Could you check a few things on this model? Use its own coordinates, in mm. A direction names the side the tool comes from. Give positions to 0.01 mm unless a question says otherwise; leave off trailing zeros. Order: outer loops, then holes, each group sorted by start corner. A loop starts at its lowest first (then second) coordinate and runs counter-clockwise, first axis right, second up. Notation, with made-up numbers: (-3.75, 35) -> (30.25, 35) arc R25 cw to (30.25, 58) -> close; hole circle Ø1 at (80.25, 31). An arc over 180 degrees is marked (long way). Write each question's results on one line, items separated by ' | '.
Autodesk Inventor part; units mm, degrees
ref_plane "YZ Plane" through (0, 0, 0) normal (1, 0, 0) x (0, 1, 0)
ref_plane "XZ Plane" through (0, 0, 0) normal (0, 1, 0) x (-1, 0, 0)
ref_plane "XY Plane" through (0, 0, 0) normal (0, 0, 1) x (1, 0, 0)
sketch "Esboço1" plane through (0, 0, 0) normal (0, 0, 1) x (1, 0, 0)
  circle A0 centre (0, 0) radius 10
  dimension "d0" = 20
extrude "Extrusão1" add sketch "Esboço1" along normal blind 38
chamfer "Chanfro1" distance 3 angle 45 1 edges at (-10, 0, 0)
sketch "Esboço3" plane through (0, 0, 0) normal (0, 1, 0) x (-1, 0, 0)
  line L0 (10, 38) -> (-10, 38)
  arc A0 (14.87, 38) -> (-14.87, 38) centre (0, 38) ccw
  line L1 (0, 52.87) -> (0, 38)
  line L2 (-14.87, 38) -> (14.87, 38)
  point P0 (0, 0)
  dimension "d7" = 29.74
revolve "Revolução1" add sketch "Esboço3" angle 360 about axis through (0, 0, 52.87) along (0, 0, -1) picked at (-6.4238, 41.8753) contours L0 L2 A0 L1
sketch "Esboço4" plane through (0, 0, 0) normal (0, 1, 0) x (-1, 0, 0)
  line L0 (-2, 57) -> (2, 57)
  line L1 (2, 57) -> (2, 41)
  line L2 (2, 41) -> (-2, 41)
  line L3 (-2, 41) -> (-2, 57)
  line L4 (7, 0) -> (-7, 0)
  point P0 (0, 0)
  point P1 (0, 0)
  dimension "d9" = 4
  dimension "d10" = 16
  dimension "d11" = 41
  dimension "d13" = 2
extrude "Extrusão2" cut sketch "Esboço4" along normal mid plane 38
properties part number "Parafuso da Valvula"
Q1. I need wall thicknesses on line 1 along Z through (x, y) = (1.5, 10.25); line 2 along Z through (x, y) = (-1, -5.75); line 3 along X through (y, z) = (4.25, 46.5). Which ranges of each line are inside material? Lowest first, please.
Here are the results:
line 1: z = 38 to 41 | line 2: z = 0 to 41 | line 3: x = -11.44 to -2, 2 to 11.44
Q2. Suppose I cut it at C-C on z = 6.5. Please give me the cut outline in (x, y).
Here are the results:
outline: circle Ø20 at (0, 0)
Q3. Thinking about a two-plate mould opening in X: for faces 4 (the conical face through (-1.56, -7.02, 0.19)), 5 (the flat face through (3, 10, 38)), 6 (the flat face through (-2, 0, 46)), which applies, +X half, -X half, draft (parallel to the pull), parting line (faces both ways), or undercut?
Here are the results:
face 4: parting line | face 5: draft | face 6: undercut
Q4. Suppose I cut it at D-D on z = 47.5. Please give me the cut outline in (x, y).
Here are the results:
outline: (-2, -11.26) -> (-2, 11.26) arc R11.44 ccw to start; (2, -11.26) arc R11.44 ccw to (2, 11.26) -> close
Q5. I'm going to push flat-ended pins straight in: pin 1 Ø1.5 at (x, z) = (-11, 10) entering from +Y; pin 2 Ø3.5 at (y, z) = (0.5, 49.5) entering from -X; pin 3 Ø2 at (x, z) = (6, 46) entering from +Y; pin 4 Ø6 at (y, z) = (5, 49.5) entering from +X. Where does each tip first touch, or does it pass through?
Here are the results:
pin 1: passes through | pin 2: stops at x = -11.22 | pin 3: stops at y = 11.84 | pin 4: stops at x = 11.41
Q6. Suppose I cut it at B-B on x = 0. Please give me the cut outline in (y, z).
Here are the results:
outline: (-14.87, 38) -> (-10, 38) -> (-10, 3) -> (-7, 0) -> (7, 0) -> (10, 3) -> (10, 38) -> (14.87, 38) arc R14.87 ccw to (14.56, 41) -> (-14.56, 41) arc R14.87 ccw to start
Q7. Suppose I cut it at A-A on y = 0. Please give me the cut outline in (x, z).
Here are the results:
outline: (-14.87, 38) -> (-10, 38) -> (-10, 3) -> (-7, 0) -> (7, 0) -> (10, 3) -> (10, 38) -> (14.87, 38) arc R14.87 ccw to (2, 52.73) -> (2, 41) -> (-2, 41) -> (-2, 52.73) arc R14.87 ccw to start
Q8. For faces 1 (the cylindrical face through (-2.17, 9.76, 20.26)), 2 (the flat face through (0, 0, 41)), 3 (the flat face through (0, 0, 0)), which set-ups out of +Z, -Z, +X, -X, +Y, -Y let a thin tool reach every point of the face, with its end or its side?
Here are the results:
face 1: -Z | face 2: +Z, +Y, -Y | face 3: -Z, +X, -X, +Y, -Y
